```python
from build123d import *

# Parameters (mm, degrees)
F0_W     = 100
F0_H     = 100
F0_R     = 1.5
F0_R_2   = 2.6
F1_DEPTH = 15
F2_DEPTH = 4
F3_SIZE  = 3


with BuildPart() as f1:
    # F0 (on Top) → F1 (new body)
    with BuildSketch(Plane.XY):
        Rectangle(F0_W, F0_H)
        Polygon((-37.75, -33.131198), (-33.75, -35.440599), (-33.75, -40.059401), (-37.75, -42.368802), (-41.75, -40.059401), (-41.75, -35.440599), align=None, mode=Mode.SUBTRACT)
        with Locations((-25, -25)):
            Circle(F0_R, mode=Mode.SUBTRACT)
        Polygon((37.75, -33.131198), (41.75, -35.440599), (41.75, -40.059401), (37.75, -42.368802), (33.75, -40.059401), (33.75, -35.440599), align=None, mode=Mode.SUBTRACT)
        with Locations((25, -25)):
            Circle(F0_R, mode=Mode.SUBTRACT)
        Polygon((-37.75, 33.131198), (-41.75, 35.440599), (-41.75, 40.059401), (-37.75, 42.368802), (-33.75, 40.059401), (-33.75, 35.440599), align=None, mode=Mode.SUBTRACT)
        with Locations((-25, 25)):
            Circle(F0_R, mode=Mode.SUBTRACT)
        with Locations((25, 25)):
            Circle(F0_R, mode=Mode.SUBTRACT)
        Polygon((37.75, 42.368802), (41.75, 40.059401), (41.75, 35.440599), (37.75, 33.131198), (33.75, 35.440599), (33.75, 40.059401), align=None, mode=Mode.SUBTRACT)
        Polygon((41.75, 35.440599), (41.75, 40.059401), (37.75, 42.368802), (33.75, 40.059401), (33.75, 35.440599), (37.75, 33.131198), align=None)
        with Locations((37.75, 37.75)):
            Circle(F0_R_2, mode=Mode.SUBTRACT)
        Polygon((-41.75, 40.059401), (-41.75, 35.440599), (-37.75, 33.131198), (-33.75, 35.440599), (-33.75, 40.059401), (-37.75, 42.368802), align=None)
        with Locations((-37.75, 37.75)):
            Circle(F0_R_2, mode=Mode.SUBTRACT)
        Polygon((-33.75, -40.059401), (-33.75, -35.440599), (-37.75, -33.131198), (-41.75, -35.440599), (-41.75, -40.059401), (-37.75, -42.368802), align=None)
        with Locations((-37.75, -37.75)):
            Circle(F0_R_2, mode=Mode.SUBTRACT)
        Polygon((41.75, -40.059401), (41.75, -35.440599), (37.75, -33.131198), (33.75, -35.440599), (33.75, -40.059401), (37.75, -42.368802), align=None)
        with Locations((37.75, -37.75)):
            Circle(F0_R_2, mode=Mode.SUBTRACT)
    extrude(amount=F1_DEPTH)

    # F0 (on Top) → F2 (cut)
    with BuildSketch(Plane.XY):
        Polygon((-41.75, 40.059401), (-41.75, 35.440599), (-37.75, 33.131198), (-33.75, 35.440599), (-33.75, 40.059401), (-37.75, 42.368802), align=None)
        with Locations((-37.75, 37.75)):
            Circle(F0_R_2, mode=Mode.SUBTRACT)
        Polygon((41.75, 35.440599), (41.75, 40.059401), (37.75, 42.368802), (33.75, 40.059401), (33.75, 35.440599), (37.75, 33.131198), align=None)
        with Locations((37.75, 37.75)):
            Circle(F0_R_2, mode=Mode.SUBTRACT)
        Polygon((41.75, -40.059401), (41.75, -35.440599), (37.75, -33.131198), (33.75, -35.440599), (33.75, -40.059401), (37.75, -42.368802), align=None)
        with Locations((37.75, -37.75)):
            Circle(F0_R_2, mode=Mode.SUBTRACT)
        Polygon((-33.75, -40.059401), (-33.75, -35.440599), (-37.75, -33.131198), (-41.75, -35.440599), (-41.75, -40.059401), (-37.75, -42.368802), align=None)
        with Locations((-37.75, -37.75)):
            Circle(F0_R_2, mode=Mode.SUBTRACT)
    extrude(amount=F2_DEPTH, mode=Mode.SUBTRACT)

    # F3
    f3_edges = [f1.edges().sort_by_distance(p)[0] for p in [
        (-26.5, 25, 15),
        (23.5, 25, 15),
        (23.5, -25, 15),
        (-26.5, -25, 15),
    ]]
    chamfer(f3_edges, length=F3_SIZE)


solid = f1.part
```
Could you check a few things on this model? Use its own coordinates, in mm. A direction names the side the tool comes from. Round coordinates to 2 decimals unless told otherwise and drop trailing zeros. Loops run counter-clockwise (first coordinate to the right, second up) from the corner with the lowest first, then second, coordinate; pieces in that order, holes last. Notation, with made-up numbers: (69, -9.75) -> (85, -9.75) arc R29 ccw to (85, 27.25) -> close; hole circle Ø4 at (47.5, 32). An arc over 180 degrees is marked (long way). One line per question, with ' | ' between items.
(1) If we section it at A-A on y = 25: List the corners of the cut face in (x, z) for me.
Model answer:
outline: (-50, 0) -> (-26.5, 0) -> (-26.5, 12) -> (-29.5, 15) -> (-50, 15) -> close; (-23.5, 0) -> (23.5, 0) -> (23.5, 12) -> (20.5, 15) -> (-20.5, 15) -> (-23.5, 12) -> close; (26.5, 0) -> (50, 0) -> (50, 15) -> (29.5, 15) -> (26.5, 12) -> close
(2) If we section it at D-D on y = 37.75: List the corners of the cut face in (x, z) for me.
Model answer:
outline: (-50, 0) -> (-41.75, 0) -> (-41.75, 4) -> (-40.35, 4) -> (-40.35, 15) -> (-50, 15) -> close; (-35.15, 4) -> (-33.75, 4) -> (-33.75, 0) -> (33.75, 0) -> (33.75, 4) -> (35.15, 4) -> (35.15, 15) -> (-35.15, 15) -> close; (40.35, 4) -> (41.75, 4) -> (41.75, 0) -> (50, 0) -> (50, 15) -> (40.35, 15) -> close
(3) Thinking about a two-plate mould opening in X: for faces 1 (the face through (-1, -50, 7)), 2 (the face through (35.722, -41.198, 1.972)), 3 (the face through (-50, -1, 7)), which applies, released by +X, released by -X, zero draft, split by the parting line, or undercut?
Model answer:
face 1: zero draft | face 2: undercut | face 3: released by -X
(4) For pin 1 Ø7 at (x, y) = (-37.75, 37.75) entering from -Z; pin 2 Ø4 at (x, y) = (25, 25) entering from +Z, each with a flat end and sliding along its axis, tell me the tip position at first contact or that it passes through.
Model answer:
pin 1: stops at z = 4 | pin 2: stops at z = 12.5
(5) If I drill on probe 1 along Y at (x, z) = (-37.75, 9); probe 2 along Y at (x, z) = (25, 6); probe 3 along X at (y, z) = (35.5, 3.5), over which ranges is the centre line in solid material (lowest first)?
Model answer:
probe 1: y = -50 to -40.35, -35.15 to 35.15, 40.35 to 50 | probe 2: y = -50 to -26.5, -23.5 to 23.5, 26.5 to 50 | probe 3: x = -50 to -41.75, -33.75 to 33.75, 41.75 to 50
(6) For faces 4 (the face through (33.75, -38, 2)), 5 (the face through (-24.241, 23.54, 12.146)), which set-ups out of +Z, -Z, +X, -X, +Y, -Y let a thin tool reach every point of the face, with its end or its side?
Model answer:
face 4: -Z | face 5: +Z
(7) If we section it at C-C on z = 2.25: Count the separate pieces of the cut face and the enclosed holes in it, and give its area (3 significant figures).
Model answer:
separate pieces: 1 | enclosed holes: 8 | area: 9,750 mm^2
